Geometry check sheet. Reference: the model listing, model coordinates, mm. A direction names the side the tool comes from. Round coordinates to 2 decimals unless told otherwise and drop trailing zeros. Order: outer loops, then holes, each group sorted by start corner. A loop starts at its lowest first (then second) coordinate and runs counter-clockwise, first axis right, second up. Notation, with made-up numbers: (34.25, 36.5) -> (72.25, 36.5) arc R28 ccw to (72.25, 72.5) -> close; hole circle Ø3 at (-35, 42.25). An arc over 180 degrees is marked (long way). Use a Markdown table: item, result. Add a question column.
Item 1: Mould release check, pull along X, two halves, no side actions. Record for faces 1 (the flat face through (2, 24, 6)), 2 (the flat face through (0, 13, 7)), 3 (the flat face through (2, 12, 0)), 4 (the flat face through (2.5, 24.5, 12)): pulls with the +X half, pulls with the -X half, needs draft (parallel to the pull), parting line crosses it, or undercut.
Item 2: Sectioned sample at C-C, the plane x = 1.6. Record the cut outline in (y, z).
Item 3: Sectioned sample at D-D, the plane z = 13.5. Record the cut outline in (x, y), and give its area (3 significant figures).
Item 4: Sectioned sample at A-A, the plane z = 6.5. Record the cut outline in (x, y), and give its area (3 significant figures).
Item 5: Gauge pin test, flat end, axial feed: pin 1 Ø0.8 at (x, y) = (2, 24.5) entering from -Z. Record the tip position at first contact, or that the pin passes through.
Item 6: Material ranges on probe 1 along Y at (x, z) = (1.45, 7.25); probe 2 along Z at (x, y) = (3.85, 14.5); probe 3 along Z at (x, y) = (3.45, 21.25), recorded low to high. Write a range as [from, to].
Item 7: Sectioned sample at B-B, the plane y = 13.5. Record the cut outline in (x, z), and give its area (3 significant figures).
Item 8: Set-up check for faces 5 (the flat face through (0.5, 24.5, 6.1)), 6 (the cylindrical face through (0.6, 12.68, 14.43)): record each of +Z, -Z, +X, -X, +Y, -Y from which the full face is reachable in a straight line by a thin tool's end or side.
from build123d import *

# Parameters (mm, degrees)
SKETCH1_W           = 15
SKETCH1_H           = 25
BOSS_EXTRUDE1_DEPTH = 5
FILLET1_R           = 2
SKETCH2_W           = 4
SKETCH2_H           = 12
CUT_EXTRUDE1_DEPTH  = 1


with BuildPart() as part:
    # Sketch1 → Boss-Extrude1 (new body)
    with BuildSketch(Plane(origin=(0, 0, 0), x_dir=(0, 0, -1), z_dir=(1, 0, 0))):
        with Locations((-7.5, 12.5)):
            Rectangle(SKETCH1_W, SKETCH1_H)
    extrude(amount=BOSS_EXTRUDE1_DEPTH)

    # Fillet1
    fillet1_edges = [part.edges().sort_by_distance(p)[0] for p in [
        (5, 12.5, 15),
        (0, 12.5, 15),
    ]]
    fillet(fillet1_edges, radius=FILLET1_R)

    # Sketch2 → Cut-Extrude1 (cut)
    with BuildSketch(Plane(origin=(0, 25, 0), x_dir=(1, 0, 0), z_dir=(0, 1, 0))):
        with Locations((2.5, -6)):
            Rectangle(SKETCH2_W, SKETCH2_H)
    extrude(amount=-CUT_EXTRUDE1_DEPTH, mode=Mode.SUBTRACT)


solid = part.part
Found:
| question | item | result |
|---|---|---|
| 1 | face 1 | undercut |
| 1 | face 2 | pulls with the -X half |
| 1 | face 3 | needs draft |
| 1 | face 4 | undercut |
| 2 | outline | (0, 0) -> (24, 0) -> (24, 12) -> (25, 12) -> (25, 14.96) -> (0, 14.96) -> close |
| 3 | outline | (0.06, 0) -> (4.94, 0) -> (4.94, 25) -> (0.06, 25) -> close |
| 3 | area | 122 mm2 |
| 4 | outline | (0, 0) -> (5, 0) -> (5, 25) -> (4.5, 25) -> (4.5, 24) -> (0.5, 24) -> (0.5, 25) -> (0, 25) -> close |
| 4 | area | 121 mm2 |
| 5 | pin 1 | stops at z = 12 |
| 6 | probe 1 | y = [0, 24] |
| 6 | probe 2 | z = [0, 14.81] |
| 6 | probe 3 | z = [0, 14.95] |
| 7 | outline | (0, 0) -> (5, 0) -> (5, 13) arc R2 ccw to (3, 15) -> (2, 15) arc R2 ccw to (0, 13) -> close |
| 7 | area | 73.3 mm2 |
| 8 | face 5 | -Z, +Y |
| 8 | face 6 | +Z, -X, +Y, -Y |
